Can you work these out from the drawing? Everything is in mm from the part's minimum corner. A direction names the side the tool comes from. Give positions to 0.01 mm unless a question says otherwise; leave off trailing zeros. Order: outer loops, then holes, each group sorted by start corner. A loop starts at its lowest first (then second) coordinate and runs counter-clockwise, first axis right, second up. Notation, with made-up numbers: (86, 28.5) - (126, 28.5) arc R20 ccw to (126, 35.5) - close; hole circle Ø11 at (1, -9.75). An arc over 180 degrees is marked (long way). Write each question's results on one line, items separated by ' | '. Start each with the question number.
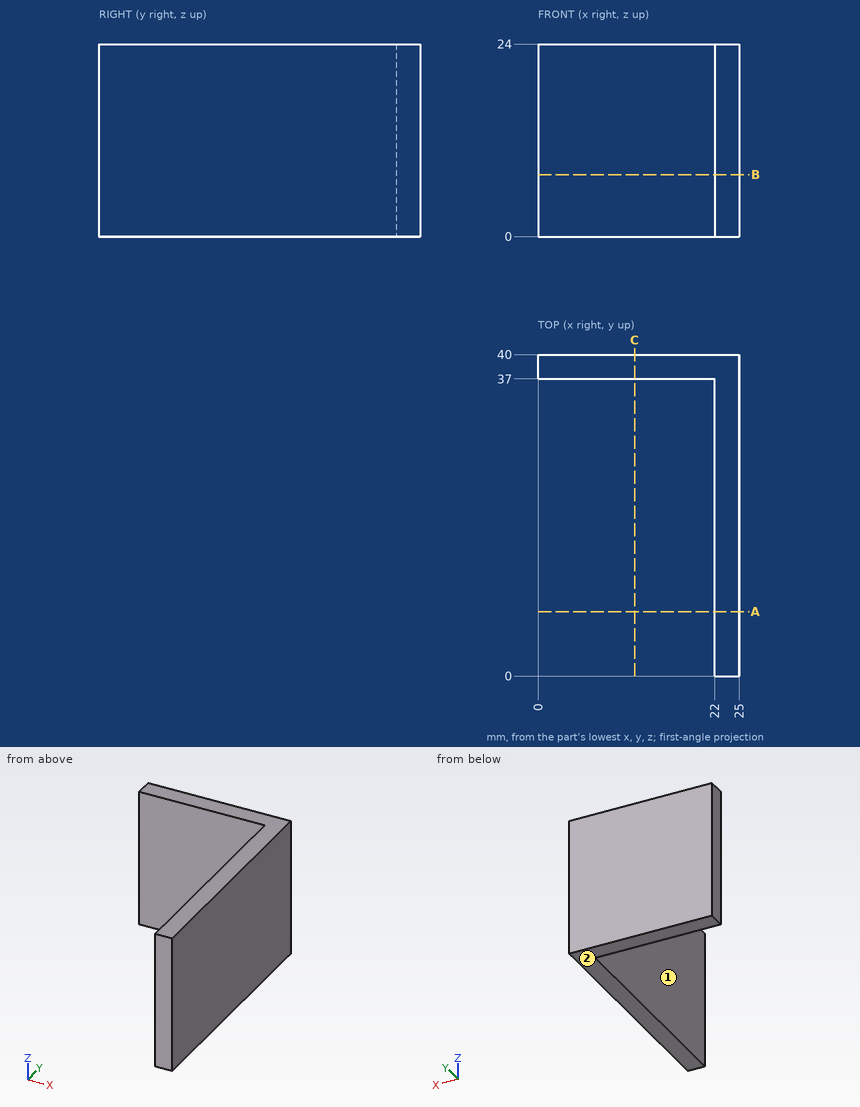
Q1. If we section it at C-C (x = 12): Please give me the cut outline in (y, z), plus the area to 3 significant figures.
Q2. Which directions (+Z, -Z, +X, -X, +Y, -Y) give clear straight access to the entire face, cutting with the end or side of a thin tool? Please do the marked faces 1 and 2.
Q3. If we section it at B-B (z = 7.75): Please give me the cut outline in (x, y), plus the area to 3 significant figures.
Q4. Will these pins go through, and if not, where does the flat tip stop? P1, Ø11, axis at x = 14.5, z = 8, coming from the -Y side; P2, Ø4, axis at y = 6.5, z = 14, coming from the -X side.
Q5. If we section it at A-A (y = 8): Please give me the cut outline in (x, z).
Q6. If I drill on probe 1 along Y at (x, z) = (20.25, 9.5); probe 2 along X at (y, z) = (19.5, 9), over which ranges is the centre line in solid material (lowest first)? Write a range as from..to.
Findings below:
1) outline: (37, 0) - (40, 0) - (40, 24) - (37, 24) - close | area: 72.0 mm2
2) face 1: +Z, -Z, -X, -Y | face 2: -Z, +X, -X, +Y, -Y
3) outline: (0, 37) - (22, 37) - (22, 0) - (25, 0) - (25, 40) - (0, 40) - close | area: 186 mm2
4) P1: stops at y = 37 | P2: stops at x = 22
5) outline: (22, 0) - (25, 0) - (25, 24) - (22, 24) - close
6) probe 1: y = 37..40 | probe 2: x = 22..25
